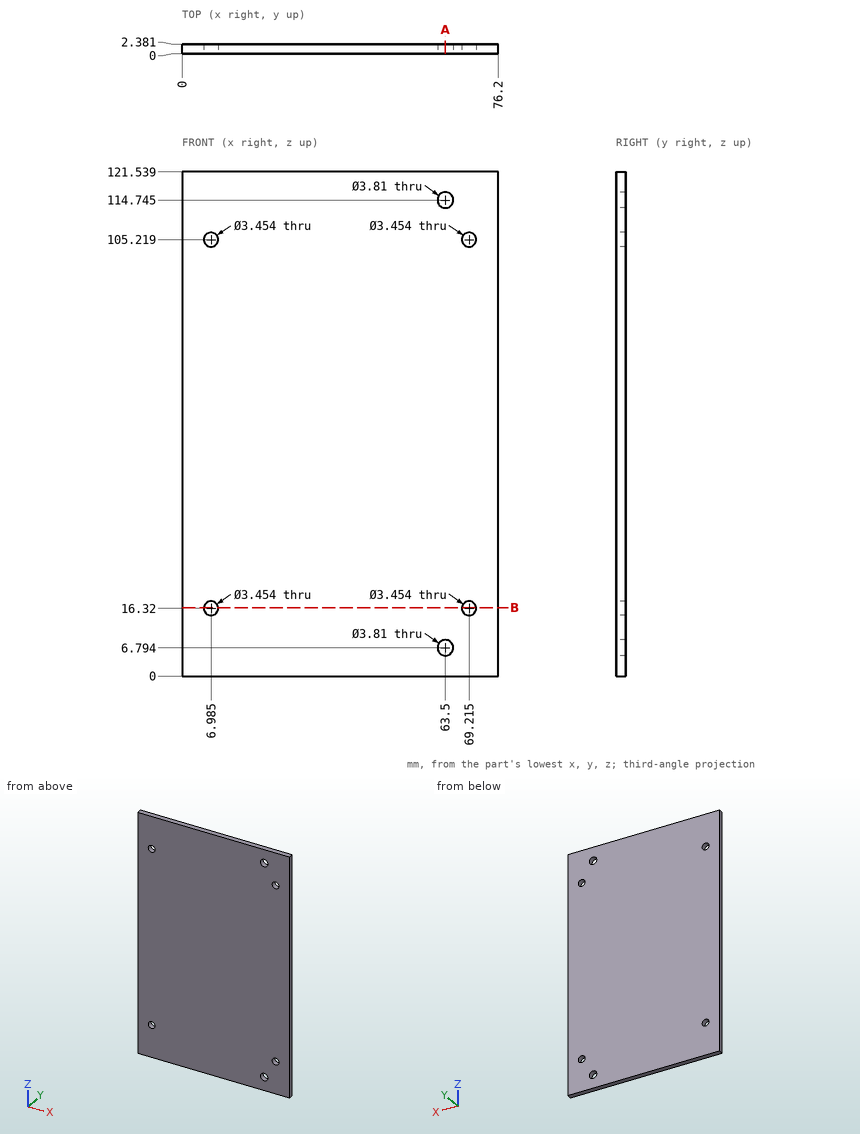
Design review of the part shown in the three views and the two pictorial views. Dimensions are in mm from the part's minimum x, y and z. Round coordinates to 2 decimals unless told otherwise and drop trailing zeros. Loops run counter-clockwise (first coordinate to the right, second up) from the corner with the lowest first, then second, coordinate; pieces in that order, holes last. Notation, with made-up numbers: (12, 4) -> (59, 4) arc R19 ccw to (59, 22) -> close; hole circle Ø5 at (-25.75, 71). An arc over 180 degrees is marked (long way). Answer as a JSON object with one key per item and string values. Group by question number.
1) For line 1 (Z direction, x = 63.5, y = 1.15); line 2 (X direction, y = 1.3, z = 17.5) (1 decimal); line 3 (X direction, y = 1.35, z = 15), list the stretches that pass through material, from the lowest coordinate up. Write a range as [from, to].
2) We need section B-B on z = 16.5. Write out the cut boundary in (x, y).
3) We need section A-A on x = 63.5. Write out the cut boundary in (y, z).
4) For pin 1 Ø4.5 at (x, z) = (63.5, 6.79) entering from +Y, flat-tipped, find the tip position at first contact; note if it passes through.
Result set:
{
 "1": {"line 1": "[0, 4.89], [8.7, 112.84], [116.65, 121.54]", "line 2": "[0, 5.7], [8.2, 68], [70.5, 76.2]", "line 3": "[0, 5.87], [8.1, 68.1], [70.33, 76.2]"},
 "2": {"outline": "(0, 0) -> (5.27, 0) -> (5.27, 2.38) -> (0, 2.38) -> close; (8.7, 0) -> (67.5, 0) -> (67.5, 2.38) -> (8.7, 2.38) -> close; (70.93, 0) -> (76.2, 0) -> (76.2, 2.38) -> (70.93, 2.38) -> close"},
 "3": {"outline": "(0, 0) -> (2.38, 0) -> (2.38, 4.89) -> (0, 4.89) -> close; (0, 8.7) -> (2.38, 8.7) -> (2.38, 112.84) -> (0, 112.84) -> close; (0, 116.65) -> (2.38, 116.65) -> (2.38, 121.54) -> (0, 121.54) -> close"},
 "4": {"pin 1": "y = 2.38"}
}
